```python
from build123d import *

# Parameters (mm, degrees)
F1_DEPTH = 25.4


with BuildPart() as f1:
    # F0 (on Front) → F1 (new body)
    with BuildSketch(Plane.XZ):
        with BuildLine():
            Line((-57.852422, -158.75), (119.170049, -158.75))
            Line((119.170049, -158.75), (119.170049, -190.5))
            Line((119.170049, -190.5), (190.290049, -190.5))
            Line((190.290049, -190.5), (190.290049, -158.75))
            Line((190.290049, -158.75), (190.290049, -127))
            Line((190.290049, -127), (0, -127))
            ThreePointArc((0, -127), (-127, 0), (0, 127))
            Line((0, 127), (153.091423, 127))
            Line((153.091423, 127), (190.290049, 127))
            Line((190.290049, 127), (190.290049, 158.75))
            Line((190.290049, 158.75), (190.290049, 190.5))
            Line((190.290049, 190.5), (119.170049, 190.5))
            Line((119.170049, 190.5), (119.170049, 158.75))
            Line((119.170049, 158.75), (-57.852422, 158.75))
            ThreePointArc((-57.852422, 158.75), (-190.290049, 0), (-57.852422, -158.75))
        make_face()
    extrude(amount=F1_DEPTH)


solid = f1.part
```
CAD build for the part. Positions are in the model's coordinates, mm. A direction names the side the tool comes from. Round coordinates to 2 decimals unless told otherwise and drop trailing zeros. Order: outer loops, then holes, each group sorted by start corner. A loop starts at its lowest first (then second) coordinate and runs counter-clockwise, first axis right, second up. Notation, with made-up numbers: (3.25, 29.25) - (44.25, 29.25) arc R36 cw to (44.25, 68.25) - close; hole circle Ø8 at (56, 30). An arc over 180 degrees is marked (long way). Answer as CSV lines item,"result". Start each with the question number.
1. Saw through at D-D, the plane z = -108. Write the cut outline in (x, y), and give its area (3 significant figures).
2. Pull direction Z, two halves, no side cores. Call faces 5 (the face through (-190.26, -12.52, 3.14)), 6 (the face through (-128, -25.4, 1)), 7 (the face through (-126.97, -12.52, -2.79)): +Z half, -Z half, draft (parallel to the pull), parting line (faces both ways), or undercut.
3. Saw through at B-B, the plane y = -5.75. Write the cut outline in (x, z), and give its area (3 significant figures).
4. Pin check, flat tips, straight feed: pin 1 (7.5 mm diameter, centred on y = -14.5, z = -172, fed in from -X); pin 2 (6 mm diameter, centred on y = -3.5, z = 61.5, fed in from -X); pin 3 (8 mm diameter, centred on y = -13, z = -25, fed in from -X). Stop position of each tip, or through.
5. Saw through at C-C, the plane z = 0. Write the cut outline in (x, y).
6. Saw through at A-A, the plane x = 31. Write the cut outline in (y, z).
7. Tool access for faces 1 (the face through (154, -13, -190.5)), 2 (the face through (29, -13, -158.75)), 3 (the face through (119.17, -13, 175)), 4 (the face through (96, -13, -127)): list every direction of +Z, -Z, +X, -X, +Y, -Y with a clear straight run to the whole face (end or side of a thin tool).
8. Drill centre lines: L1, parallel to Z at x = 36, y = -2.75; L2, parallel to Z at x = 133, y = -12.5; L3, parallel to X at y = -11.25, z = 168.5. Where is each one in solid material? Low to high. Write a range as [from, to].
Model answer:
1,outline,"(-148.82, -25.4) - (-66.82, -25.4) - (-66.82, 0) - (-148.82, 0) - close"
1,area,"2,080 mm²"
2,face 5,"parting line"
2,face 6,"draft"
2,face 7,"undercut"
3,outline,"(-57.85, -158.75) - (119.17, -158.75) - (119.17, -190.5) - (190.29, -190.5) - (190.29, -127) - (0, -127) arc R127 cw to (0, 127) - (190.29, 127) - (190.29, 190.5) - (119.17, 190.5) - (119.17, 158.75) - (-57.85, 158.75) arc R161.36 ccw to start"
3,area,"41,200 mm²"
4,pin 1,"stops at x = 119.17"
4,pin 2,"stops at x = -179.31"
4,pin 3,"stops at x = -188.92"
5,outline,"(-190.29, -25.4) - (-127, -25.4) - (-127, 0) - (-190.29, 0) - close"
6,outline,"(-25.4, -158.75) - (0, -158.75) - (0, -127) - (-25.4, -127) - close; (-25.4, 127) - (0, 127) - (0, 158.75) - (-25.4, 158.75) - close"
7,face 1,"-Z, +X, -X, +Y, -Y"
7,face 2,"-Z, -X, +Y, -Y"
7,face 3,"+Z, -X, +Y, -Y"
7,face 4,"+X, +Y, -Y"
8,L1,"z = [-158.75, -127], [127, 158.75]"
8,L2,"z = [-190.5, -127], [127, 190.5]"
8,L3,"x = [119.17, 190.29]"
